```python
from build123d import *

# Parameters (mm, degrees)
SKETCH_1_R      = 0.4
EXTRUDE_1_DEPTH = 0.7


with BuildPart() as part:
    # 草图1 → 凸台-拉伸1 (new body)
    with BuildSketch(Plane.XY):
        with BuildLine():
            Line((-0.25, -2.336664289), (-0.25, -4.736664289))
            Line((-0.25, -4.736664289), (-0.55, -4.736664289))
            ThreePointArc((-0.55, -4.736664289), (-1.398077663, -4.385642662), (-1.749999324, -3.537938086))
            ThreePointArc((-1.749999324, -3.537938086), (-1.933378352, -2.344928231), (-2.464284459, -1.260936032))
            ThreePointArc((-2.464284459, -1.260936032), (0, 3.45), (2.464284459, -1.260936032))
            ThreePointArc((2.464284459, -1.260936032), (1.933378352, -2.344928231), (1.749999324, -3.537938086))
            ThreePointArc((1.749999324, -3.537938086), (1.398077663, -4.385642662), (0.55, -4.736664289))
            Line((0.55, -4.736664289), (0.25, -4.736664289))
            Line((0.25, -4.736664289), (0.25, -2.336664289))
            ThreePointArc((0.25, -2.336664289), (0, 2.35), (-0.25, -2.336664289))
        make_face()
        with Locations(Location((-1.05, -3.736664289, 0), (0, 0, 180))):
            Circle(SKETCH_1_R, mode=Mode.SUBTRACT)
        with Locations((1.05, -3.736664289)):
            Circle(SKETCH_1_R, mode=Mode.SUBTRACT)
    extrude(amount=EXTRUDE_1_DEPTH)


solid = part.part
```
Verification items for the finished model (mm, model axes). Give positions to 0.01 mm unless a question says otherwise; leave off trailing zeros. Order: outer loops, then holes, each group sorted by start corner. A loop starts at its lowest first (then second) coordinate and runs counter-clockwise, first axis right, second up. Notation, with made-up numbers: (46.5, 79.5) - (52.5, 79.5) arc R13 cw to (52.5, 84.5) - close; hole circle Ø10 at (45, 16). An arc over 180 degrees is marked (long way). Answer as CSV lines item,"result". Start each with the question number.
Item 1: Section check D-D, the plane x = -1.25. Record the boundary of the cut face in (y, z), plus the area to 3 significant figures.
Item 2: Section check C-C, the plane z = 0.2. Record the boundary of the cut face in (x, y), plus the area to 3 significant figures.
Item 3: Gauge pin test, flat end, axial feed: pin 1 (3 mm diameter, centred on x = 2.5, y = 1, fed in from -Z). Record the tip position at first contact, or that the pin passes through.
Item 4: Mould release check, pull along Y, two halves, no side actions. Record for faces 1 (the face through (-1.389, -4.395, 0.345)), 2 (the face through (-0.09, 3.45, 0.35)), 3 (the face through (-0.998, -4.133, 0.345)): released by +Y, released by -Y, zero draft, split by the parting line, or undercut.
Item 5: Material ranges on L1, parallel to Y at x = 1.05, z = 0.5; L2, parallel to X at y = -4, z = 0.4; L3, parallel to X at y = -3.5, z = 0.6, recorded low to high.
Item 6: Section check B-B, the plane y = 0. Record the boundary of the cut face in (x, z).
Item 7: Section check A-A, the plane x = 1. Record the boundary of the cut face in (y, z), plus the area to 3 significant figures.
Filled in:
1,outline,"(-4.51, 0) - (-4.08, 0) - (-4.08, 0.7) - (-4.51, 0.7) - close; (-3.39, 0) - (-1.99, 0) - (-1.99, 0.7) - (-3.39, 0.7) - close; (1.99, 0) - (3.18, 0) - (3.18, 0.7) - (1.99, 0.7) - close"
1,area,"2.11 mm^2"
2,outline,"(-2.46, -1.26) arc R4 cw to (-1.75, -3.54) arc R1.2 ccw to (-0.55, -4.74) - (-0.25, -4.74) - (-0.25, -2.34) arc R2.35 cw (long way) to (0.25, -2.34) - (0.25, -4.74) - (0.55, -4.74) arc R1.2 ccw to (1.75, -3.54) arc R4 cw to (2.46, -1.26) arc R3 ccw (long way) to start; hole circle Ø0.8 at (-1.05, -3.74); hole circle Ø0.8 at (1.05, -3.74)"
2,area,"16.9 mm^2"
3,pin 1,"z = 0"
4,face 1,"released by -Y"
4,face 2,"split by the parting line"
4,face 3,"undercut"
5,L1,"-4.63 to -4.14, -3.34 to -2.1, 2.1 to 3.26"
5,L2,"-1.66 to -1.35, -0.75 to -0.25, 0.25 to 0.75, 1.35 to 1.66"
5,L3,"-1.75 to -1.37, -0.73 to -0.25, 0.25 to 0.73, 1.37 to 1.75"
6,outline,"(-2.97, 0) - (-2.35, 0) - (-2.35, 0.7) - (-2.97, 0.7) - close; (2.35, 0) - (2.97, 0) - (2.97, 0.7) - (2.35, 0.7) - close"
7,outline,"(-4.65, 0) - (-4.13, 0) - (-4.13, 0.7) - (-4.65, 0.7) - close; (-3.34, 0) - (-2.13, 0) - (-2.13, 0.7) - (-3.34, 0.7) - close; (2.13, 0) - (3.28, 0) - (3.28, 0.7) - (2.13, 0.7) - close"
7,area,"2.02 mm^2"
